from build123d import *

# Parameters (mm, degrees)
EXTRUDE_1_DEPTH     = 4.7
CUT_EXTRUDE_START   = -1.5
CUT_EXTRUDE_1_DEPTH = 1.5
CUT_EXTRUDE_2_DEPTH = 1.5
CUT_EXTRUDE_3_DEPTH = 8.192704637
FILLET_1_R          = 0.2


with BuildPart() as part:
    # 草图1 → 凸台-拉伸1 (new body)
    with BuildSketch(Plane.XY):
        with BuildLine():
            Line((-1.4, -3.586432768), (-1.4, -1.428285686))
            ThreePointArc((-1.4, -1.428285686), (0, 2), (1.4, -1.428285686))
            Line((1.4, -1.428285686), (1.4, -3.586432768))
            ThreePointArc((1.4, -3.586432768), (0, 3.85), (-1.4, -3.586432768))
        make_face()
    extrude(amount=EXTRUDE_1_DEPTH)

    # 草图2 → 切除-拉伸1 (cut)
    with BuildSketch(Plane.XY.offset(4.7).offset(CUT_EXTRUDE_START)):
        with BuildLine():
            Line((-0.5, 1.936491673), (-0.5, 3.817394399))
            ThreePointArc((-0.5, 3.817394399), (0, 3.85), (0.5, 3.817394399))
            Line((0.5, 3.817394399), (0.5, 1.936491673))
            ThreePointArc((0.5, 1.936491673), (0, 2), (-0.5, 1.936491673))
        make_face()
    extrude(amount=CUT_EXTRUDE_1_DEPTH, mode=Mode.SUBTRACT)

    # 草图3 → 切除-拉伸2 (cut)
    with BuildSketch(Plane(origin=(0, 0, 0), x_dir=(-1, 0, 0), z_dir=(0, 0, -1))):
        with BuildLine():
            Line((-1.767766953, -1.767766953), (-2.474873734, -2.474873734))
            ThreePointArc((-2.474873734, -2.474873734), (0, 3.5), (2.474873734, -2.474873734))
            Line((2.474873734, -2.474873734), (1.767766953, -1.767766953))
            ThreePointArc((1.767766953, -1.767766953), (0, 2.5), (-1.767766953, -1.767766953))
        make_face()
    extrude(amount=-CUT_EXTRUDE_2_DEPTH, mode=Mode.SUBTRACT)

    # 草图4 → 切除-拉伸3 (cut, through all)
    with BuildSketch(Plane(origin=(0, 0, 0), x_dir=(-1, 0, 0), z_dir=(0, 0, -1))):
        with BuildLine():
            Line((-0.5, 1.936491673), (-0.5, 2.244994432))
            ThreePointArc((-0.5, 2.244994432), (0, 2.3), (0.5, 2.244994432))
            Line((0.5, 2.244994432), (0.5, 1.936491673))
            ThreePointArc((0.5, 1.936491673), (0, 2), (-0.5, 1.936491673))
        make_face()
    extrude(amount=-CUT_EXTRUDE_3_DEPTH, mode=Mode.SUBTRACT)

    # 圆角1
    fillet_1_edges = [part.edges().sort_by_distance(p)[0] for p in [
        (-1.932079623, 0.516786543, 4.7),
        (1.4, -2.507359227, 4.7),
        (-3.821866583, 0.464581337, 4.7),
        (1.932079623, 0.516786543, 4.7),
        (0.5, 2.876943036, 4.7),
        (-0.5, 2.876943036, 4.7),
        (3.821866583, 0.464581337, 4.7),
        (0, 3.85, 0),
        (-1.4, -2.507359227, 4.7),
        (1.4, -3.586432768, 2.35),
        (-1.4, -3.586432768, 2.35),
    ]]
    fillet(fillet_1_edges, radius=FILLET_1_R)


solid = part.part
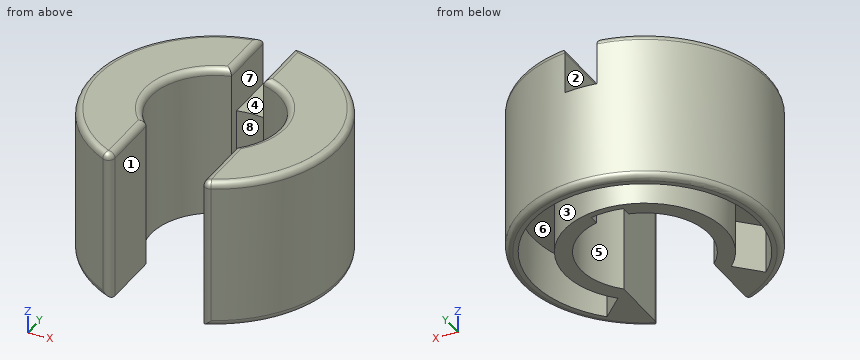
Geometry check sheet. Reference: the model listing, model coordinates, mm. Face numbers are marked on the shaded views. A direction names the side the tool comes from. Give positions to 0.01 mm unless a question says otherwise; leave off trailing zeros. Order: outer loops, then holes, each group sorted by start corner. A loop starts at its lowest first (then second) coordinate and runs counter-clockwise, first axis right, second up.
1) Draft check along Y on the marked faces 6, 7 and 8. Enter one of: released by +Y, released by -Y, zero draft, split by the parting line, or undercut.
Results are:
face 6: undercut
face 7: zero draft
face 8: released by -Y
2) Gauge pin test, flat ends, axial feed: pin 1 (1.5 mm diameter, centred on y = -2.5, z = 2, fed in from -X); pin 2 (0.6 mm diameter, centred on y = -2, z = 2, fed in from +X); pin 3 (2 mm diameter, centred on y = 3, z = 1.5, fed in from -X). Record the tip position at first contact, or that the pin passes through.
Results are:
pin 1: stops at x = -3.43
pin 2: stops at x = 3.45
pin 3: stops at x = -3.29
3) Cross-section at A-A (z = 4.1). Record the boundary of the cut face in (x, y), then the cut area to 3 significant figures.
Results are:
outline: (-1.69, -3.46) arc R0.2 ccw to (-1.4, -3.28) - (-1.4, -1.43) arc R2 cw to (-0.5, 1.94) - (-0.5, 3.82) arc R3.85 ccw to start; (0.5, 1.94) arc R2 cw to (1.4, -1.43) - (1.4, -3.28) arc R0.2 ccw to (1.69, -3.46) arc R3.85 ccw to (0.5, 3.82) - close
area: 26.7 mm2
4) Tool access check on the marked faces 1, 2, 3, 4 and 5. Record the directions out of +Z, -Z, +X, -X, +Y, -Y that give a thin tool (end or side, any length) a straight path to the whole face; none if there is none.
Results are:
face 1: +Z, -Z, -Y
face 2: +Z, -Y
face 3: -Z
face 4: +Z, +Y, -Y
face 5: +Z, -Z
5) Material ranges on probe 1 along X at (y, z) = (0, 0.5); probe 2 along Y at (x, z) = (0, 0.45); probe 3 along Y at (x, z) = (0.75, 0.8), recorded low to high.
Results are:
probe 1: x = -3.85 to -3.5, -2.5 to -2, 2 to 2.5, 3.5 to 3.85
probe 2: y = 2.3 to 2.5, 3.5 to 3.85
probe 3: y = 1.85 to 2.38, 3.42 to 3.78
6) Cross-section at C-C (x = 0). Record the boundary of the cut face in (y, z), then the cut area to 3 significant figures.
Results are:
outline: (2.3, 0) - (2.5, 0) - (2.5, 1.5) - (3.5, 1.5) - (3.5, 0) - (3.65, 0) arc R0.2 ccw to (3.85, 0.2) - (3.85, 3.2) - (2.3, 3.2) - close
area: 3.45 mm2
